Model file for the job. Use its own axes, mm. A direction names the side the tool comes from. Coordinates: 2 decimals unless noted, no trailing zeros. Loops run counter-clockwise (first coordinate to the right, second up) from the corner with the lowest first, then second, coordinate; pieces in that order, holes last. Notation, with made-up numbers: M 24,21.25 L 29,21.25 A25 cw 29,42.25 Z; hole C 66,85 d5. An arc over 180 degrees is marked long. Write item = value, one per line. Start each with the question number.
from build123d import *

# Parameters (mm, degrees)
F0_W     = 37
F0_H     = 15
F1_DEPTH = 450
F2_W     = 31
F2_H     = 444
F3_DEPTH = 12
F4_R     = 2
F5_DEPTH = 450.001
F6_R     = 1
F7_R     = 1


with BuildPart() as f1:
    # F0 (on Top) → F1 (new body)
    with BuildSketch(Plane.XY):
        Rectangle(F0_W, F0_H)
    extrude(amount=F1_DEPTH)

    # F2 (on face) → F3 (cut)
    with BuildSketch(Plane(origin=(0, 7.5, 0), x_dir=(-1, 0, 0), z_dir=(0, 1, 0))):
        with Locations((0, 225)):
            Rectangle(F2_W, F2_H)
    extrude(amount=-F3_DEPTH, mode=Mode.SUBTRACT)

    # F4 (on face) → F5 (cut, through all)
    with BuildSketch(Plane.XY.offset(450)):
        with Locations((9, 0)):
            Circle(F4_R)
        with Locations((-9, 0)):
            Circle(F4_R)
    extrude(amount=-F5_DEPTH, mode=Mode.SUBTRACT)

    # F6
    f6_edges = [f1.edges().sort_by_distance(p)[0] for p in [
        (-18.5, 0, 450),
        (18.5, 0, 450),
        (-18.5, 0, 0),
        (18.5, 0, 0),
    ]]
    fillet(f6_edges, radius=F6_R)

    # F7
    f7_edges = [f1.edges().sort_by_distance(p)[0] for p in [
        (18.5, -7.5, 225),
        (18.5, 7.5, 225),
    ]]
    fillet(f7_edges, radius=F7_R)


solid = f1.part
Item 1: Pin check, flat tips, straight feed: pin 1 Ø3 at (x, y) = (-9, 0) entering from -Z; pin 2 Ø5 at (x, z) = (10, 221) entering from +Y; pin 3 Ø4.5 at (x, y) = (-9, 0) entering from -Z. Stop position of each tip, or through.
Item 2: 3-axis set-ups, long thin cutter, end or side, ignore diameter. For faces 1 (the flat face through (0, 0, 450)), 2 (the flat face through (15.5, 2, 222)): which of +Z, -Z, +X, -X, +Y, -Y reach the whole face in a straight line?
Item 3: Probe L1, parallel to Y at x = 9, z = 1.9; L2, parallel to X at y = 2.25, z = 362; L3, parallel to Z at x = -13, y = 5. List the from-to ranges inside material, lowest first.
Item 4: Cut at A-A (z = 285). Give the cut face in (x, y), plus the area to 3 significant figures.
Reported:
q1.pin_1 = through
q1.pin_2 = -4.5
q1.pin_3 = 0
q2.face_1 = +Z, +X, -X, +Y, -Y
q2.face_2 = +Y
q3.L1 = -7.5 to -2, 2 to 7.5
q3.L2 = -18.5 to -15.5, 15.5 to 18.5
q3.L3 = 0 to 3, 447 to 450
q4.outline = M -18.5,-6.5 A1 ccw -17.5,-7.5 L 17.5,-7.5 A1 ccw 18.5,-6.5 L 18.5,6.5 A1 ccw 17.5,7.5 L 15.5,7.5 L 15.5,-4.5 L -15.5,-4.5 L -15.5,7.5 L -17.5,7.5 A1 ccw -18.5,6.5 Z
q4.area = 182 mm^2
